Autodesk Inventor part; units mm, degrees
ref_plane "YZ Plane" through (0, 0, 0) normal (1, 0, 0) x (0, 1, 0)
ref_plane "XZ Plane" through (0, 0, 0) normal (0, 1, 0) x (-1, 0, 0)
ref_plane "XY Plane" through (0, 0, 0) normal (0, 0, 1) x (1, 0, 0)
sketch "スケッチ1" plane through (0, 0, 0) normal (0, 0, 1) x (1, 0, 0)
  circle A0 centre (0, 0) radius 50
  dimension "d0" = 100
extrude "押し出し1" add sketch "スケッチ1" along normal blind 60
sketch "スケッチ2" plane through (0, 0, 60) normal (0, 0, 1) x (1, 0, 0)
  point P0 (0, 0)
  point P1 (0, 0)
hole "穴1" at (0, 0, 60) direction (0, 0, -1) diameter 10 depth 60 tip angle 118
sketch "スケッチ3" plane through (0, 0, 60) normal (0, 0, 1) x (1, 0, 0)
  circle A0 centre (0, 0) radius 5
  circle A1 centre (0, 0) radius 10 construction
  point P0 (-9.9993, 0.1214)
  point P1 (-0.1795, 9.9984)
  point P2 (9.997, -0.246)
  dimension "d17" = 20
hole "穴2" at (-9.9993, 0.1214, 60) at (-0.1795, 9.9984, 60) at (9.997, -0.246, 60) direction (0, 0, -1) diameter 5 depth 60 tip angle 118
properties part number "ローラー"
Verification items for the finished model (mm, model axes). Give positions to 0.01 mm unless a question says otherwise; leave off trailing zeros. Loops run counter-clockwise (first coordinate to the right, second up) from the corner with the lowest first, then second, coordinate; pieces in that order, holes last. Notation, with made-up numbers: (-14, -16) - (21, -16) arc R19 cw to (21, 18) - close; hole circle Ø5 at (63, -33). An arc over 180 degrees is marked (long way). Write item = value, one per line. Start each with the question number.
Q1. Depth check by flat-ended pin: P1, Ø2, axis at x = -19, z = 40.5, coming from the -Y side; P2, Ø8, axis at x = 36, z = 24.5, coming from the +Y side; P3, Ø2, axis at y = -4.5, z = 52, coming from the -X side. Enter the tip coordinate at first touch or a pass-through.
Q2. Cross-section at B-B, the plane z = 20.5. Enter the section's corners in (x, y), and give its area (3 significant figures).
Q3. Mould release check, pull along Y, two halves, no side actions. Record for faces 1 (the face through (47.69, -15.02, 29.58)), 2 (the face through (4.88, 1.08, 29.58)), 3 (the face through (-1, -10, 0)): released by +Y, released by -Y, zero draft, split by the parting line, or undercut.
Q4. Cross-section at A-A, the plane y = 0. Enter the section's corners in (x, z).
Q5. Cross-section at C-C, the plane x = 21. Enter the section's corners in (y, z), and give its area (3 significant figures).
Q6. Cross-section at D-D, the plane y = 24. Enter the section's corners in (x, z), and give its area (3 significant figures).
Q7. Thickness scan on line 1 (X direction, y = -2, z = 20); line 2 (Y direction, x = 2.5, z = 4); line 3 (X direction, y = 10.5, z = 15.5). Record the ranges inside material, lowest first.
Answer key:
q1.P1 = -46.65
q1.P2 = 38.42
q1.P3 = -49.88
q2.outline = circle Ø100 at (0, 0); hole circle Ø5 at (-10, 0.12); hole circle Ø10 at (0, 0); hole circle Ø5 at (-0.18, 10); hole circle Ø5 at (10, -0.25)
q2.area = 7,720 mm^2
q3.face_1 = split by the parting line
q3.face_2 = undercut
q3.face_3 = zero draft
q4.outline = (-50, 0) - (-12.5, 0) - (-12.5, 60) - (-50, 60) - close; (-7.5, 0) - (-5, 0) - (-5, 60) - (-7.5, 60) - close; (5, 0) - (7.51, 0) - (7.51, 60) - (5, 60) - close; (12.48, 0) - (50, 0) - (50, 60) - (12.48, 60) - close
q5.outline = (-45.38, 0) - (45.38, 0) - (45.38, 60) - (-45.38, 60) - close
q5.area = 5,450 mm^2
q6.outline = (-43.86, 0) - (43.86, 0) - (43.86, 60) - (-43.86, 60) - close
q6.area = 5,260 mm^2
q7.line_1 = -49.96 to -11.32, -8.68 to -4.58, 4.58 to 8.22, 11.78 to 49.96
q7.line_2 = -49.94 to -4.33, 4.33 to 49.94
q7.line_3 = -48.89 to -2.63, 2.27 to 48.89
